The listing builds one solid part. Answer for the finished solid, in the listing's coordinates (mm). Coordinates: 2 decimals unless noted, no trailing zeros. Use one line per item in the form item = value. Start each with the question number.
```python
from build123d import *
from OCP.BRepAlgoAPI import BRepAlgoAPI_Cut
from OCP.TopTools import TopTools_ListOfShape

# Parameters (mm, degrees)
SKETCH1_W           = 158
SKETCH1_H           = 308
SKETCH1_R           = 1.5
SKETCH1_R_2         = 3
BOSS_EXTRUDE1_DEPTH = 12
SKETCH5_R           = 3
CUT_EXTRUDE4_DEPTH  = 3
CUT_EXTRUDE4_TAPER  = 45
CUT_EXTRUDE5_START  = 103.536585
SKETCH6_R           = 1.5
CUT_EXTRUDE5_DEPTH  = 20


with BuildPart() as part:
    # Sketch1 → Boss-Extrude1 (new body)
    with BuildSketch(Plane.XY):
        with Locations((-77.951219512, -50.463414634)):
            Rectangle(SKETCH1_W, SKETCH1_H)
        with Locations((-129.951219512, -28.463414634)):
            Circle(SKETCH1_R, mode=Mode.SUBTRACT)
        with Locations((-25.951219512, -28.463414634)):
            Circle(SKETCH1_R, mode=Mode.SUBTRACT)
        with Locations((-34.951219512, 40.536585366)):
            Circle(SKETCH1_R, mode=Mode.SUBTRACT)
        with Locations((-4.951219512, -184.463414634)):
            Circle(SKETCH1_R, mode=Mode.SUBTRACT)
        with Locations((-4.951219512, -56.463414634)):
            Circle(SKETCH1_R, mode=Mode.SUBTRACT)
        with Locations((-150.951219512, -184.463414634)):
            Circle(SKETCH1_R, mode=Mode.SUBTRACT)
        with Locations((-150.951219512, -56.463414634)):
            Circle(SKETCH1_R, mode=Mode.SUBTRACT)
        with Locations((-120.951219512, 40.536585366)):
            Circle(SKETCH1_R_2, mode=Mode.SUBTRACT)
    extrude(amount=BOSS_EXTRUDE1_DEPTH)

    # Sketch5 → Cut-Extrude4 (cut)
    with BuildSketch(Plane.XY):
        with Locations((-25.951219512, -28.463414634)):
            Circle(SKETCH5_R)
        with Locations((-129.951219512, -28.463414634)):
            Circle(SKETCH5_R)
        with Locations((-34.951219512, 40.536585366)):
            Circle(SKETCH5_R)
        with Locations((-4.951219512, -56.463414634)):
            Circle(SKETCH5_R)
        with Locations((-4.951219512, -184.463414634)):
            Circle(SKETCH5_R)
        with Locations((-150.951219512, -56.463414634)):
            Circle(SKETCH5_R)
        with Locations((-150.951219512, -184.463414634)):
            Circle(SKETCH5_R)
    extrude(amount=CUT_EXTRUDE4_DEPTH, taper=CUT_EXTRUDE4_TAPER, mode=Mode.SUBTRACT)


with BuildPart() as cut_extrude5_tool:
    # Sketch6 → Cut-Extrude5 (new body)
    with BuildSketch(Plane(origin=(0, 0, 0), x_dir=(1, 0, 0), z_dir=(0, 1, 0)).offset(CUT_EXTRUDE5_START)):
        with Locations(Location((-141.951219512, -6, 0), (0, 0, 90))):
            Circle(SKETCH6_R)
        with Locations(Location((-13.951219512, -6, 0), (0, 0, 90))):
            Circle(SKETCH6_R)
    extrude(amount=-CUT_EXTRUDE5_DEPTH)


with BuildPart() as part_1:
    add(part.part)

    # Cut-Extrude5: cut by cut_extrude5_tool, with a tolerance
    cut_extrude5_stock = TopTools_ListOfShape()
    cut_extrude5_stock.Append(part_1.part.wrapped)
    cut_extrude5_tools = TopTools_ListOfShape()
    cut_extrude5_tools.Append(cut_extrude5_tool.part.wrapped)
    cut_extrude5_cut = BRepAlgoAPI_Cut()
    cut_extrude5_cut.SetArguments(cut_extrude5_stock)
    cut_extrude5_cut.SetTools(cut_extrude5_tools)
    cut_extrude5_cut.SetFuzzyValue(0.00001)
    cut_extrude5_cut.Build()
    add(Compound.cast(cut_extrude5_cut.Shape()).solids(), mode=Mode.REPLACE)


solid = part_1.part
```
(1) Determine the mould class of faces 1 (the face through (-118.09, 41.44, 5.92)), 2 (the face through (1.049, -53, 6)), 3 (the face through (-79, -48, 12)), 4 (the face through (-156.951, -53, 6)) for opening direction X: +X half, -X half, draft (parallel to the pull), parting line (faces both ways), or undercut.
(2) Find the intervals of material crossed by probe 1 along X at (y, z) = (96.75, 6); probe 2 along X at (y, z) = (39.5, 2), in increasing order. Write a range as from..to.
(3) Each of these flat-tipped pins is pushed along its axis until it touches: pin 1 Ø3.5 at (x, y) = (-4.95, -184.46) entering from -Z; pin 2 Ø5 at (x, y) = (-150.95, -184.46) entering from -Z. Where does it stop, or does it pass through?
Evaluation:
q1.face_1 = undercut
q1.face_2 = +X half
q1.face_3 = draft
q1.face_4 = -X half
q2.probe_1 = -156.95..-143.45, -140.45..-15.45, -12.45..1.05
q2.probe_2 = -156.95..-123.77, -118.14..-36.04, -33.87..1.05
q3.pin_1 = 1.25
q3.pin_2 = 0.5
